```python
from build123d import *

# Parameters (mm, degrees)
SKETCH2_W           = 76.2
SKETCH2_H           = 76.2
SKETCH2_W_2         = 73.66
SKETCH2_H_2         = 73.66
BOSS_EXTRUDE1_DEPTH = 203.2
SKETCH3_W           = 73.66
SKETCH3_H           = 73.66
BOSS_EXTRUDE2_DEPTH = 1.27


with BuildPart() as part:
    # Sketch2 → Boss-Extrude1 (new body)
    with BuildSketch(Plane(origin=(0, 0, 0), x_dir=(1, 0, 0), z_dir=(0, 1, 0))):
        Rectangle(SKETCH2_W, SKETCH2_H)
        Rectangle(SKETCH2_W_2, SKETCH2_H_2, mode=Mode.SUBTRACT)
    extrude(amount=BOSS_EXTRUDE1_DEPTH)

    # Sketch3 → Boss-Extrude2 (add)
    with BuildSketch(Plane(origin=(0, 203.2, 0), x_dir=(1, 0, 0), z_dir=(0, 1, 0))):
        Rectangle(SKETCH3_W, SKETCH3_H)
    extrude(amount=-BOSS_EXTRUDE2_DEPTH)


solid = part.part
```
Input: part model. Units: mm. Frame: model coordinates. A direction names the side the tool comes from. Coordinates: 2 decimals unless noted, no trailing zeros. Loops run counter-clockwise (first coordinate to the right, second up) from the corner with the lowest first, then second, coordinate; pieces in that order, holes last. Notation, with made-up numbers: M 23,85.5 L 68,85.5 A23 ccw 68,95.5 Z; hole C 15.5,-4.75 d8. An arc over 180 degrees is marked long. Answer in a Markdown table with one row per item.
1. Draft query along Z for faces 3 (the flat face through (-1, 100, 38.1)), 4 (the flat face through (-1, 100, -38.1)), 5 (the flat face through (-1, 100, -36.83)), 6 (the flat face through (38.1, 100, 1)). Return one class per face: pulls with the +Z half, pulls with the -Z half, needs draft (parallel to the pull), parting line crosses it, or undercut.
Response:
| item | result |
|---|---|
| face 3 | pulls with the +Z half |
| face 4 | pulls with the -Z half |
| face 5 | undercut |
| face 6 | needs draft |
2. Section B-B, the plane x = -4. Output: boundary loops of the cut face in (y, z), then the cut area to 3 significant figures.
Response:
| item | result |
|---|---|
| outline | M 0,-38.1 L 203.2,-38.1 L 203.2,38.1 L 0,38.1 L 0,36.83 L 201.93,36.83 L 201.93,-36.83 L 0,-36.83 Z |
| area | 610 mm2 |
3. Section C-C, the plane z = -24. Output: boundary loops of the cut face in (x, y).
Response:
| item | result |
|---|---|
| outline | M -38.1,0 L -36.83,0 L -36.83,201.93 L 36.83,201.93 L 36.83,0 L 38.1,0 L 38.1,203.2 L -38.1,203.2 Z |
4. First-contact query: pin 1 (4 mm diameter, centred on x = 20, z = -21.5, fed in from -Y). Flat tip, straight axial feed; report the tip coordinate or a pass-through.
Response:
| item | result |
|---|---|
| pin 1 | stops at y = 201.93 |
5. Section A-A, the plane y = 15. Output: boundary loops of the cut face in (x, z).
Response:
| item | result |
|---|---|
| outline | M -38.1,-38.1 L 38.1,-38.1 L 38.1,38.1 L -38.1,38.1 Z; hole M -36.83,-36.83 L 36.83,-36.83 L 36.83,36.83 L -36.83,36.83 Z |
6. Material intervals for line 1 (Z direction, x = -9, y = 15); line 2 (Y direction, x = 9, z = -0.5), sorted ascending.
Response:
| item | result |
|---|---|
| line 1 | z = -38.1 to -36.83, 36.83 to 38.1 |
| line 2 | y = 201.93 to 203.2 |
7. Reachability of faces 1 (the flat face through (-1, 203.2, -1)), 2 (the flat face through (-36.83, 100, 1)) from +Z, -Z, +X, -X, +Y, -Y: full face, straight path, thin tool, end or side. Return the list, or none.
Response:
| item | result |
|---|---|
| face 1 | +Z, -Z, +X, -X, +Y |
| face 2 | -Y |
